For this review, take the finished solid that the model builds, in its own axes (mm). Face numbers are marked on the shaded views. A direction names the side the tool comes from. Coordinates: 2 decimals unless noted, no trailing zeros. Order: outer loops, then holes, each group sorted by start corner. A loop starts at its lowest first (then second) coordinate and runs counter-clockwise, first axis right, second up.
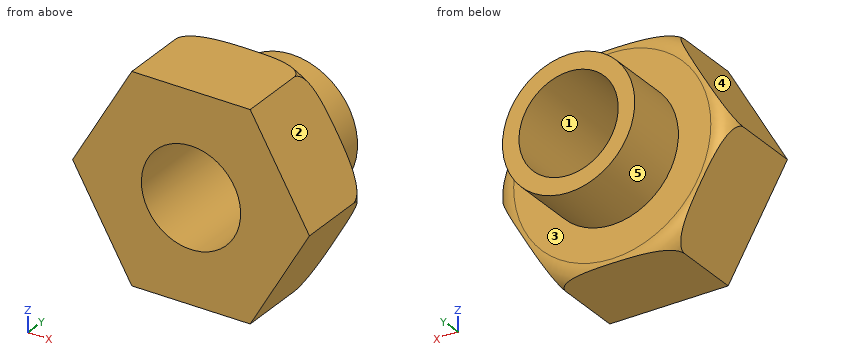
from build123d import *

# Parameters (mm, degrees)
BOSS_EXTRUDE1_DEPTH     = 65
SKETCH4_R               = 50
BOSS_EXTRUDE2_DEPTH     = 50
CUT_EXTRUDE1_DEPTH      = 166.044186174
CUT_EXTRUDE1_DEPTH_BACK = 166.044186174
SKETCH5_R               = 37.5


with BuildPart() as part:
    # Sketch1 → Boss-Extrude1 (new body)
    with BuildSketch(Plane(origin=(0, 0, 0), x_dir=(1, 0, 0), z_dir=(0, 1, 0))):
        Polygon((-44.744645862, -77.5), (44.744645862, -77.5), (89.489291724, 0), (-89.489291724, 0), align=None)
        Polygon((-89.489291724, 0), (89.489291724, 0), (44.744645862, 77.5), (-44.744645862, 77.5), align=None)
    extrude(amount=BOSS_EXTRUDE1_DEPTH)

    # Sketch2 → Cut-Revolve1 (revolve, cut)
    with BuildSketch(Plane.XY, mode=Mode.PRIVATE) as cut_revolve1_sk:
        with BuildLine():
            Line((74.489291724, 65), (74.489291724, 71.033853329))
            Line((74.489291724, 71.033853329), (95.90922918, 71.033853329))
            Line((95.90922918, 71.033853329), (95.90922918, 50))
            Line((95.90922918, 50), (89.489291724, 50))
            ThreePointArc((89.489291724, 50), (85.095893442, 60.606601718), (74.489291724, 65))
        make_face()
    revolve(cut_revolve1_sk.sketch.rotate(Axis((0, 0, 0), (0, 1, 0)), 90), axis=Axis((0, 0, 0), (0, 1, 0)), mode=Mode.SUBTRACT)

    # Sketch4 → Boss-Extrude2 (add)
    with BuildSketch(Plane(origin=(0, 65, 0), x_dir=(1, 0, 0), z_dir=(0, 1, 0))):
        with Locations(Location((0, 0, 0), (0, 0, 270))):
            Circle(SKETCH4_R)
    extrude(amount=BOSS_EXTRUDE2_DEPTH)

    # Sketch5 → Cut-Extrude1 (cut, two sides: drawn at the far end of the back side and taken through both)
    with BuildSketch(Plane(origin=(0, 115, 0), x_dir=(1, 0, 0), z_dir=(0, 1, 0)).offset(-CUT_EXTRUDE1_DEPTH_BACK)):
        with Locations(Location((0, 0, 0), (0, 0, 270))):
            Circle(SKETCH5_R)
    extrude(amount=CUT_EXTRUDE1_DEPTH + CUT_EXTRUDE1_DEPTH_BACK, mode=Mode.SUBTRACT)


solid = part.part
1. The part is to be moulded in two halves that separate along Z. For the marked faces 1, 2 and 3, say which applies: +Z half, -Z half, draft (parallel to the pull), parting line (faces both ways), or undercut.
Answer below:
face 1: undercut
face 2: +Z half
face 3: draft
2. Take a section at A-A, the plane y = 41. Give the boundary of the cut face in (x, z), plus the area to 3 significant figures.
Answer below:
outline: (-89.49, 0) - (-44.74, -77.5) - (44.74, -77.5) - (89.49, 0) - (44.74, 77.5) - (-44.74, 77.5) - close; hole circle Ø75 at (0, 0)
area: 16,400 mm2
3. Take a section at C-C, the plane y = 93. Give the boundary of the cut face in (x, z), plus the area to 3 significant figures.
Answer below:
outline: circle Ø100 at (0, 0); hole circle Ø75 at (0, 0)
area: 3,440 mm2
4. Machinability: for the marked faces 4 and 5, which of the approach directions +Z, -Z, +X, -X, +Y, -Y give a long, thin tool a straight path to every point of the face, cutting with its end or side? Answer none if there is none.
Answer below:
face 4: +Z, -X, +Y, -Y
face 5: +Y
5. Clearance check with flat-ended pins moving along their axes: pin 1 Ø4 at (y, z) = (45.5, 3.5) entering from +X; pin 2 Ø1.5 at (x, y) = (-65.5, 25.5) entering from -Z; pin 3 Ø1 at (y, z) = (54.5, -18.5) entering from -X. State where each tip first meets the part, or that it passes through.
Answer below:
pin 1: stops at x = 88.62
pin 2: stops at z = -42.85
pin 3: stops at x = -79.1
6. Take a section at B-B, the plane y = 53.5. Give the boundary of the cut face in (x, z), plus the area to 3 significant figures.
Answer below:
outline: (-89.07, -0.72) - (-45.16, -76.78) arc R89.08 ccw to (-43.91, -77.5) - (43.91, -77.5) arc R89.08 ccw to (45.16, -76.78) - (89.07, -0.72) arc R89.08 ccw to (89.07, 0.72) - (45.16, 76.78) arc R89.08 ccw to (43.91, 77.5) - (-43.91, 77.5) arc R89.08 ccw to (-45.16, 76.78) - (-89.07, 0.72) arc R89.08 ccw to start; hole circle Ø75 at (0, 0)
area: 16,400 mm2
7. To check wall thickness, follow L1, parallel to X at y = 72, z = 0; L2, parallel to X at y = 29.5, z = 0; L3, parallel to Y at x = 53, z = 22. State the ranges of each line that lie inside material, in increasing order.
Answer below:
L1: x = -50 to -37.5, 37.5 to 50
L2: x = -89.49 to -37.5, 37.5 to 89.49
L3: y = 0 to 65
